Verification items for the finished model (mm, model axes). A direction names the side the tool comes from. Round coordinates to 2 decimals unless told otherwise and drop trailing zeros. Order: outer loops, then holes, each group sorted by start corner. A loop starts at its lowest first (then second) coordinate and runs counter-clockwise, first axis right, second up. Notation, with made-up numbers: (57, -8.75) -> (106, -8.75) arc R27 cw to (106, 16.25) -> close; hole circle Ø10 at (88, 22.5). An arc over 180 degrees is marked (long way). Return JSON: item names as keys, results as strings. Group by question number.
Item 1: Sectioned sample at A-A on z = 14.45. Record the cut outline in (x, y), plus the area to 3 significant figures.
Item 2: Scan lines: probe 1 along Z at (x, y) = (11.1, -1.75); probe 2 along X at (y, z) = (19.25, 23.25). Record each from-to range of solid material in increasing order. Write a range as from..to.
Item 3: Access from +Z, -Z, +X, -X, +Y, -Y to the whole of each face (thin tool, end or side, straight path). Record for faces 1 (the flat face through (22.2, -2, 14)), 2 (the flat face through (11, 0, 11)).
Item 4: Sectioned sample at D-D on z = 24.25. Record the cut outline in (x, y).
Item 5: Draft check along Y on faces 3 (the flat face through (-3.2, 7, 14)), 4 (the flat face through (-1.6, 21.2, 1)), 5 (the cylindrical face through (-1.578, 8.103, 14.582)). Enter one of: pulls with the +Y half, pulls with the -Y half, needs draft (parallel to the pull), parting line crosses it, or undercut.
Item 6: Sectioned sample at B-B on x = 11.1. Record the cut outline in (y, z).
Item 7: Depth check by flat-ended pin: pin 1 Ø6 at (x, z) = (11, 15.5) entering from +Y; pin 2 Ø5 at (y, z) = (17, 3.5) entering from +X. Enter the tip coordinate at first touch or a pass-through.
```python
from build123d import *

# Parameters (mm, degrees)
RESSALTO_EXTRUS_O1_DEPTH = 28.9
CHANFRO1_SIZE            = 2
ESBO_O2_R                = 3
CORTE_EXTRUS_O1_DEPTH    = 43.671887701
ESBO_O3_R                = 3
CORTE_EXTRUS_O2_DEPTH    = 43.671887701


with BuildPart() as part:
    # Esboço1 → Ressalto-extrusão1 (new body)
    with BuildSketch(Plane.XY):
        Polygon((0, 0), (0, 22.2), (-3.2, 22.2), (-3.2, -3.2), (22.2, -3.2), (22.2, 0), align=None)
    extrude(amount=RESSALTO_EXTRUS_O1_DEPTH)

    # Chanfro1
    chanfro1_edges = [part.edges().sort_by_distance(p)[0] for p in [
        (-1.6, 22.2, 28.9),
        (22.2, -1.6, 28.9),
        (22.2, -1.6, 0),
        (-1.6, 22.2, 0),
    ]]
    chamfer(chanfro1_edges, length=CHANFRO1_SIZE)

    # Esboço2 → Corte-extrusão1 (cut, through all)
    with BuildSketch(Plane(origin=(0, 0, 0), x_dir=(1, 0, 0), z_dir=(0, 1, 0))):
        with Locations(Location((11.1, -14.45, 0), (0, 0, 180))):
            Circle(ESBO_O2_R)
    extrude(amount=-CORTE_EXTRUS_O1_DEPTH, mode=Mode.SUBTRACT)

    # Esboço3 → Corte-extrusão2 (cut, through all)
    with BuildSketch(Plane(origin=(0, 0, 0), x_dir=(0, 0, -1), z_dir=(1, 0, 0))):
        with Locations(Location((-14.45, 11.1, 0), (0, 0, 90))):
            Circle(ESBO_O3_R)
    extrude(amount=-CORTE_EXTRUS_O2_DEPTH, mode=Mode.SUBTRACT)


solid = part.part
```
Recorded:
{
 "1": {"outline": "(-3.2, -3.2) -> (8.1, -3.2) -> (8.1, 0) -> (0, 0) -> (0, 8.1) -> (-3.2, 8.1) -> close; (-3.2, 14.1) -> (0, 14.1) -> (0, 22.2) -> (-3.2, 22.2) -> close; (14.1, -3.2) -> (22.2, -3.2) -> (22.2, 0) -> (14.1, 0) -> close", "area": "114 mm²"},
 "2": {"probe 1": "0..11.45, 17.45..28.9", "probe 2": "-3.2..0"},
 "3": {"face 1": "+Z, -Z, +X, +Y, -Y", "face 2": "+Z, -Z, +X, +Y"},
 "4": {"outline": "(-3.2, -3.2) -> (22.2, -3.2) -> (22.2, 0) -> (0, 0) -> (0, 22.2) -> (-3.2, 22.2) -> close"},
 "5": {"face 3": "needs draft", "face 4": "pulls with the +Y half", "face 5": "undercut"},
 "6": {"outline": "(-3.2, 0) -> (0, 0) -> (0, 11.45) -> (-3.2, 11.45) -> close; (-3.2, 17.45) -> (0, 17.45) -> (0, 28.9) -> (-3.2, 28.9) -> close"},
 "7": {"pin 1": "y = 0", "pin 2": "x = 0"}
}
